from build123d import *

# Parameters (mm, degrees)
CROQUIS1_W              = 500
CROQUIS1_H              = 260
SALIENTE_EXTRUIR1_DEPTH = 3
CROQUIS2_W              = 30
CROQUIS2_H              = 30
CORTAR_EXTRUIR1_DEPTH   = 4
CORTAR_EXTRUIR2_DEPTH   = 4


with BuildPart() as part:
    # Croquis1 → Saliente-Extruir1 (new body)
    with BuildSketch(Plane.XY):
        Rectangle(CROQUIS1_W, CROQUIS1_H)
    extrude(amount=SALIENTE_EXTRUIR1_DEPTH)

    # Croquis2 → Cortar-Extruir1 (cut, through all)
    with BuildSketch(Plane.XY.offset(3)):
        with Locations((-80, 115)):
            Rectangle(CROQUIS2_W, CROQUIS2_H)
        with Locations((-235, 115)):
            Rectangle(CROQUIS2_W, CROQUIS2_H)
    cortar_extruir1 = extrude(amount=-CORTAR_EXTRUIR1_DEPTH, mode=Mode.SUBTRACT)

    # Simetría1: Cortar-Extruir1 across plane
    add(cortar_extruir1.mirror(Plane(origin=(0, 0, 0), x_dir=(0, 0, 1), z_dir=(1, 0, 0))), mode=Mode.SUBTRACT)

    # Croquis3 → Cortar-Extruir2 (cut, through all)
    with BuildSketch(Plane.XY.offset(3)):
        Polygon((-250, -130), (-240, -130), (-240, 120), (0, 120), (0, 130), (-240, 130), (-250, 130), align=None)
    cortar_extruir2 = extrude(amount=-CORTAR_EXTRUIR2_DEPTH, mode=Mode.SUBTRACT)

    # Simetría2: Cortar-Extruir2 across plane
    add(cortar_extruir2.mirror(Plane(origin=(0, 0, 0), x_dir=(0, 0, 1), z_dir=(1, 0, 0))), mode=Mode.SUBTRACT)


solid = part.part
Work out the finished part from the listing and answer in its coordinate system (mm). Round coordinates to 2 decimals unless told otherwise and drop trailing zeros. Write each loop counter-clockwise with the first axis right and the second up, starting at its lowest first coordinate (ties: lowest second). Pieces come first, ordered by that corner, then holes. Notation, with made-up numbers: M 29,66 L 59,66 A30 ccw 59,91 Z; hole C 29,-33 d9. An arc over 180 degrees is marked long. Use a Markdown table: item, result.
1) Flat-ended cylindrical pins translate along their axes: pin 1 (1.5 mm diameter, centred on y = 110, z = 2, fed in from -X); pin 2 (0.9 mm diameter, centred on y = 107.5, z = 2, fed in from +X); pin 3 (1.5 mm diameter, centred on x = 75, z = 1, fed in from +Y). Find the tip coordinate at first contact, or state that the pin passes through.
Taken from the geometry:
| item | result |
|---|---|
| pin 1 | stops at x = -220 |
| pin 2 | stops at x = 220 |
| pin 3 | stops at y = 100 |
2) The part is cut by section B-B on x = -82. Give the vertices of the cut face in (y, z), plus the area to 3 significant figures.
Taken from the geometry:
| item | result |
|---|---|
| outline | M -130,0 L 100,0 L 100,3 L -130,3 Z |
| area | 690 mm2 |
3) The part is cut by section A-A on z = 1.65. Give the vertices of the cut face in (x, y).
Taken from the geometry:
| item | result |
|---|---|
| outline | M -240,-130 L 240,-130 L 240,100 L 220,100 L 220,120 L 95,120 L 95,100 L 65,100 L 65,120 L -65,120 L -65,100 L -95,100 L -95,120 L -220,120 L -220,100 L -240,100 Z |
4) Consider line 1 (Y direction, x = 89, z = 2.5). Determine where the line is inside the solid, lowest interval first. Write a range as [from, to].
Taken from the geometry:
| item | result |
|---|---|
| line 1 | y = [-130, 100] |
